Drawing for the job (mm, zero at the part's lowest x, y, z). Round coordinates to 2 decimals unless told otherwise and drop trailing zeros. Loops run counter-clockwise (first coordinate to the right, second up) from the corner with the lowest first, then second, coordinate; pieces in that order, holes last. Notation, with made-up numbers: (64, -28) -> (100, -28) arc R11 ccw to (100, -20) -> close; hole circle Ø2 at (-16, -26). An arc over 180 degrees is marked (long way). Put each result on its own line as item: value. Start each with the question number.
Item 1: Cut at C-C, the plane y = 13. Count the separate pieces of the cut face and the enclosed holes in it, plus the area to 3 significant figures.
Item 2: Cut at A-A, the plane x = 50.8. List the corners of the cut face in (y, z).
Item 3: Flat gauge pins, fed straight in: pin 1 Ø4 at (y, z) = (21.5, 24.5) entering from -X; pin 2 Ø10 at (x, y) = (67, 8.5) entering from +Z; pin 3 Ø1.5 at (x, y) = (52, 8.5) entering from +Z. Where does each tip first touch, or does it go through?
Item 4: Cut at D-D, the plane x = 62. List the corners of the cut face in (y, z), plus the area to 3 significant figures.
Item 5: Pull direction X, two halves, no side cores. Call the marked faces 1, 2 and 3: +X half, -X half, draft (parallel to the pull), parting line (faces both ways), or undercut.
Item 6: Drill centre lines: probe 1 along X at (y, z) = (1.5, 60); probe 2 along X at (y, z) = (10.75, 60.5) (1 decimal); probe 3 along X at (y, z) = (14.75, 83.5) (1 decimal). Where is each one in solid material? Low to high. Write a range as [from, to].
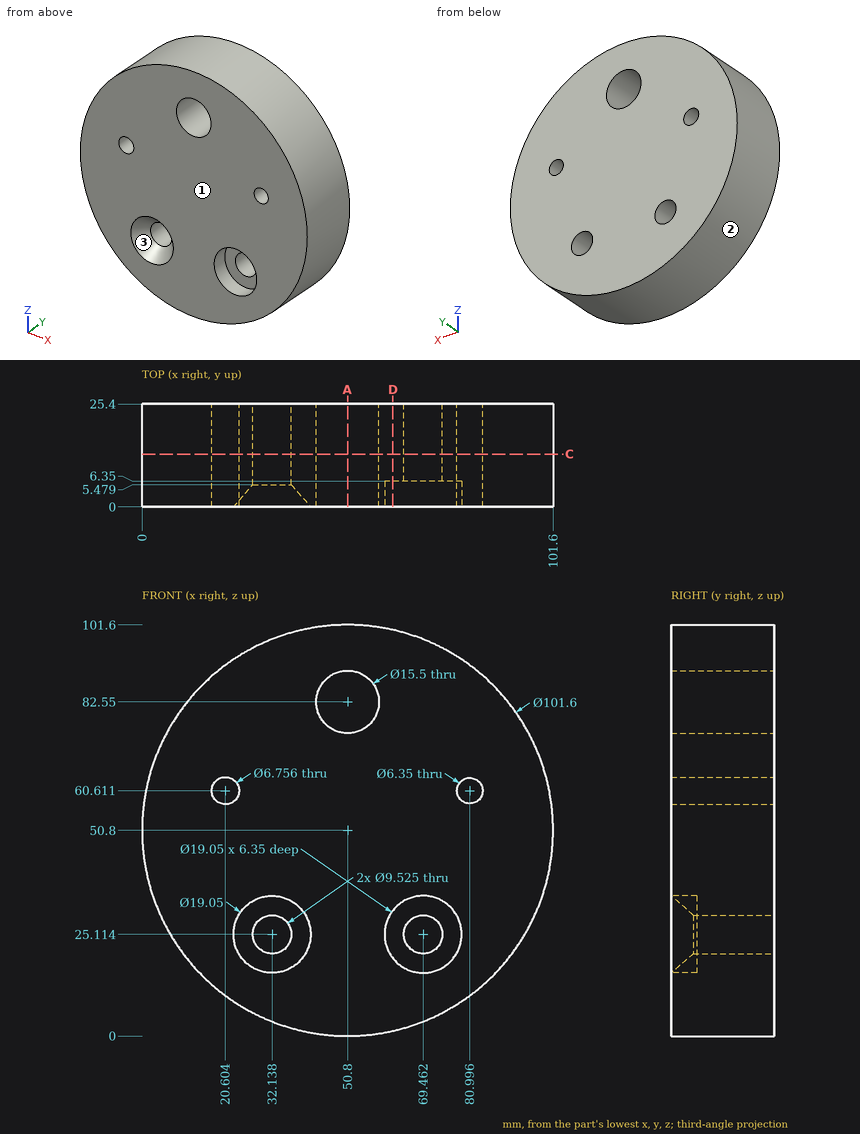
Reply:
1. separate pieces: 1
1. enclosed holes: 5
1. area: 7,710 mm^2
2. outline: (0, 0) -> (25.4, 0) -> (25.4, 74.8) -> (0, 74.8) -> close; (0, 90.3) -> (25.4, 90.3) -> (25.4, 101.6) -> (0, 101.6) -> close
3. pin 1: stops at x = 6.19
3. pin 2: stops at z = 100.35
3. pin 3: stops at z = 101.6
4. outline: (0, 1.25) -> (25.4, 1.25) -> (25.4, 100.35) -> (0, 100.35) -> (0, 31.03) -> (6.35, 31.03) -> (6.35, 19.19) -> (0, 19.19) -> close
4. area: 2,440 mm^2
5. face 1: draft
5. face 2: parting line
5. face 3: undercut
6. probe 1: x = [0.84, 17.28], [23.93, 77.88], [84.11, 100.76]
6. probe 2: x = [0.9, 17.2], [24, 77.8], [84.2, 100.7]
6. probe 3: x = [11.9, 43.1], [58.5, 89.7]
